Model file for the job. Use its own axes, mm. A direction names the side the tool comes from. Give positions to 0.01 mm unless a question says otherwise; leave off trailing zeros. Loops run counter-clockwise (first coordinate to the right, second up) from the corner with the lowest first, then second, coordinate; pieces in that order, holes last. Notation, with made-up numbers: (6, -34.5) -> (38, -34.5) arc R31 ccw to (38, 2.5) -> close; hole circle Ø8 at (57.5, 67). An arc over 180 degrees is marked (long way). Use CSV: the item, a comma, the result in double quotes. Start each with the question number.
(1) Cut at D-D on z = -4. Write the cut outline in (x, y), then the cut area to 3 significant figures.
(2) Drill centre lines: probe 1 along Y at (x, z) = (51, -73); probe 2 along Z at (x, y) = (93.5, -24.5); probe 3 along Y at (x, z) = (31.5, -62). Where is each one in solid material? Low to high.
(3) 3-axis set-ups, long thin cutter, end or side, ignore diameter. For faces 4 (the flat face through (84, 92.026, -81)), 5 (the flat face through (84, 95.026, -87)), 6 (the cylindrical face through (81.345, 86.727, -35.29)), 7 (the flat face through (81, -26, 67.215)), 8 (the cylindrical face through (128.417, -32.233, 65.738)): which of +Z, -Z, +X, -X, +Y, -Y reach the whole face in a straight line?
(4) Cut at C-C on y = -25. Write the cut outline in (x, z), then the cut area to 3 significant figures.
(5) Pull direction X, two halves, no side cores. Call faces 1 (the cylindrical face through (81.34, 88.77, -32.99)), 2 (the cylindrical face through (37.42, 93.546, -89.047)), 3 (the flat face through (0, 67, -15)): pulls with the +X half, pulls with the -X half, needs draft (parallel to the pull), parting line crosses it, or undercut.
(6) Cut at A-A on x = 40. State how many separate pieces and enclosed holes the cut face has, then the cut area to 3 significant figures.
(7) Flat gauge pins, fed straight in: pin 1 (4 mm diameter, centred on x = 25.5, y = 50, fed in from -Z); pin 2 (10 mm diameter, centred on x = 120, z = -85, fed in from +Y); pin 3 (3 mm diameter, centred on x = 104.5, z = -71.5, fed in from +Y); pin 4 (3.5 mm diameter, centred on x = 74, y = 96.5, fed in from -Z). Where does each tip first touch, or does it go through?
Solid Edge part; units mm, degrees
sketch "Sketch1" plane through (0, 0, 0) normal (1, 0, 0) x (0, 1, 0)
  arc A0 (2.0255, 64.2182) -> (12.0255, 54.2182) centre (2.0255, 54.2182) cw
  arc A1 (12.0255, 54.2182) -> (62.1552, -15.4154) centre (85.1165, 53.9757) ccw
  arc A2 (62.1552, -15.4154) -> (95.0255, -66.6818) centre (43.6001, -63.4831) cw
  line L0 (95.0255, -66.6818) -> (95.0255, -76.6818)
  line L1 (95.0255, -76.6818) -> (98.0468, -76.6818)
  line L2 (98.0468, -76.6818) -> (98.0468, -65.8944)
  arc A3 (62.6354, -12.4154) -> (98.0468, -65.8944) centre (43.6001, -63.4831) cw
  arc A4 (15.0228, 54.2182) -> (62.6354, -12.4154) centre (85.1165, 53.9757) ccw
  arc A5 (2.0255, 67.2155) -> (15.0228, 54.2182) centre (2.0255, 54.2182) cw
  line L3 (2.0255, 64.2182) -> (2.0255, 67.2155)
  dimension "D1" = 95.0255
  dimension "D2" = 2.0255
extrude "Protrusion1" add sketch "Sketch1" along normal blind 165
sketch "Sketch2" plane through (75, 2.0255, 65.7168) normal (0, -1, 0) x (1, 0, 0)
  line L0 (-75, 1.4986) -> (90, 1.4986)
  line L1 (90, 1.4986) -> (90, -1.4986)
  line L2 (90, -1.4986) -> (-75, -1.4986)
  line L3 (-75, -1.4986) -> (-75, 1.4986)
extrude "Extrusionsausprägung_2" add sketch "Sketch2" along normal blind 56
sketch "Sketch3" plane through (82.5, -22.9745, 67.2155) normal (0, 0, 1) x (0, 1, 0)
  circle A0 centre (-8.5, 42.5) radius 3.5
  circle A1 centre (-8.5, -42.5) radius 3.5
extrude "Cutout1" cut sketch "Sketch3" against normal through all
sketch "Sketch4" plane through (165, 28.0437, -4.7332) normal (1, 0, 0) x (0, 1, 0)
  line L0 (66.9818, -61.9486) -> (63.9818, -61.9486)
  line L1 (63.9818, -61.9486) -> (63.9818, -91.9486)
  line L2 (63.9818, -91.9486) -> (66.9818, -91.9486)
  line L3 (66.9818, -91.9486) -> (66.9818, -61.9486)
  dimension "D1" = 66.9818
  dimension "D2" = 63.9818
extrude "Protrusion2" add sketch "Sketch4" against normal up to vertex (165 mm away)
sketch "Sketch5" plane through (82.5, 95.0255, -86.6818) normal (0, 1, 0) x (1, 0, 0)
  circle A0 centre (-42.5, 0) radius 3.5
  circle A1 centre (42.5, 0) radius 3.5
  dimension "D1" = 42.5
extrude "Cutout2" cut sketch "Sketch5" against normal through all
properties material "Nylon, allgemein"
Check result:
1,outline,"(0, 40.61) -> (165, 40.61) -> (165, 45.72) -> (0, 45.72) -> close"
1,area,"844 mm²"
2,probe 1,"92.03 to 98.05"
2,probe 2,"64.22 to 67.22"
2,probe 3,"95.1 to 98.08"
3,face 4,"-Z, +X, -X, -Y"
3,face 5,"-Z, +X, -X, +Y"
3,face 6,"+X, -X, -Y"
3,face 7,"+Z, +X, -X, +Y, -Y"
3,face 8,"+Z, -Z"
4,outline,"(0, 64.22) -> (165, 64.22) -> (165, 67.22) -> (0, 67.22) -> close"
4,area,"495 mm²"
5,face 1,"needs draft"
5,face 2,"undercut"
5,face 3,"pulls with the -X half"
6,separate pieces,"3"
6,enclosed holes,"0"
6,area,"769 mm²"
7,pin 1,"z = -11.18"
7,pin 2,"y = 95.03"
7,pin 3,"y = 98.05"
7,pin 4,"z = -96.68"
